Could you check a few things on this model? Use its own coordinates, in mm. A direction names the side the tool comes from. Coordinates: 2 decimals unless noted, no trailing zeros. Loops run counter-clockwise (first coordinate to the right, second up) from the corner with the lowest first, then second, coordinate; pieces in that order, holes last. Notation, with made-up numbers: M 12,-19 L 47,-19 A25 cw 47,4 Z; hole C -2,-33 d7. An arc over 180 degrees is marked long. Return JSON: item names as keys, results as strings. Group by question number.
from build123d import *

# Parameters (mm, degrees)
BOSS_EXTRUDE1_START      = -1
SKETCH1_W                = 1.7
SKETCH1_H                = 89.2
BOSS_EXTRUDE1_DEPTH      = 8.8
SKETCH4_W                = 33.7
SKETCH4_H                = 11.6
BOSS_EXTRUDE3_DEPTH      = 8.8
SERVO_HOLDER_DEPTH       = 1
SERVO_HOLDER_DEPTH_BACK  = 8.8
SKETCH3_W                = 14
SKETCH3_H                = 7
SKETCH3_R                = 1
SKETCH37_W               = 20
SKETCH37_H               = 7
BOSS_EXTRUDE19_DEPTH     = 9.8
CUT_EXTRUDE10_DEPTH      = 93.434679639
CUT_EXTRUDE10_DEPTH_BACK = 93.434679639
SKETCH29_W               = 34.409909993
SKETCH29_H               = 6.377389624
BOSS_EXTRUDE13_START     = 2
SKETCH30_W               = 34
SKETCH30_H               = 38
SKETCH30_R               = 1.6
BOSS_EXTRUDE13_DEPTH     = 6.5
SKETCH41_W               = 17.288461538
SKETCH41_H               = 8.8
CUT_EXTRUDE14_DEPTH      = 15
BOSS_EXTRUDE14_START     = -38
SKETCH32_R               = 1.45
SKETCH32_R_2             = 5
BOSS_EXTRUDE14_DEPTH     = 8.8
BOSS_EXTRUDE16_DEPTH     = 3
BOSS_EXTRUDE17_DEPTH     = 3
BOSS_EXTRUDE18_DEPTH     = 8.8
SKETCH39_W               = 1.7
SKETCH39_H               = 41.2
BOSS_EXTRUDE20_DEPTH     = 8.8
CUT_EXTRUDE13_DEPTH      = 17.5
CHAMFER2_SIZE            = 0.6
CHAMFER2_SIZE_2          = 1.039230485
CHAMFER3_SIZE            = 3
FILLET10_R               = 6
CUT_EXTRUDE15_DEPTH      = 10
CHAMFER4_SIZE            = 2.5
CUT_EXTRUDE16_DEPTH      = 10
FILLET11_R               = 0.8
SKETCH44_W               = 59.192885725
SKETCH44_H               = 45.417181718
CUT_EXTRUDE17_DEPTH      = 87.948983376


with BuildPart() as part:
    # Sketch1 → Boss-Extrude1 (new body)
    with BuildSketch(Plane(origin=(0, 0, 0), x_dir=(1, 0, 0), z_dir=(0, 1, 0)).offset(BOSS_EXTRUDE1_START)):
        with Locations((-20.85, 25.311538462)):
            Rectangle(SKETCH1_W, SKETCH1_H)
    extrude(amount=-BOSS_EXTRUDE1_DEPTH)

    # Sketch4 → Boss-Extrude3 (add)
    with BuildSketch(Plane.XZ.offset(9.8)):
        with Locations((-4.85, -64.111538462)):
            Rectangle(SKETCH4_W, SKETCH4_H)
    extrude(amount=-BOSS_EXTRUDE3_DEPTH)

    # Sketch3 → Servo Holder (add, two sides: drawn at the far end of the back side and taken through both)
    # profile 1 of 2: a face of its own
    with BuildSketch(Plane.XZ.offset(9.8).offset(-SERVO_HOLDER_DEPTH_BACK)):
        with Locations((-14.7, -55.411538462)):
            Rectangle(SKETCH3_W, SKETCH3_H)
        with Locations(Location((-14, -54.311538462, 0), (0, 0, 270))):
            Circle(SKETCH3_R, mode=Mode.SUBTRACT)
    # profile 2 of 2: a face of its own
    with BuildSketch(Plane.XZ.offset(9.8).offset(-SERVO_HOLDER_DEPTH_BACK)):
        with Locations((-14.7, -25.211538462)):
            Rectangle(SKETCH3_W, SKETCH3_H)
        with Locations(Location((-14, -26.311538462, 0), (0, 0, 90))):
            Circle(SKETCH3_R, mode=Mode.SUBTRACT)
    extrude(amount=SERVO_HOLDER_DEPTH + SERVO_HOLDER_DEPTH_BACK)

    # Sketch37 → Boss-Extrude19 (add)
    with BuildSketch(Plane(origin=(0, -1, 0), x_dir=(1, 0, 0), z_dir=(0, 1, 0))):
        with Locations((2.3, 25.211538462)):
            Rectangle(SKETCH37_W, SKETCH37_H)
    extrude(amount=-BOSS_EXTRUDE19_DEPTH)

    # Sketch29 → Cut-Extrude10 (cut, two sides: drawn at the far end of the back side and taken through both)
    with BuildSketch(Plane(origin=(0, 0, -69.911538462), x_dir=(-1, 0, 0), z_dir=(0, 0, -1)).offset(-CUT_EXTRUDE10_DEPTH_BACK)):
        with Locations((4.495045004, -12.988694812)):
            Rectangle(SKETCH29_W, SKETCH29_H)
    extrude(amount=CUT_EXTRUDE10_DEPTH + CUT_EXTRUDE10_DEPTH_BACK, mode=Mode.SUBTRACT)


with BuildPart() as body_2:
    # Sketch30 → Boss-Extrude13 (new body)
    with BuildSketch(Plane.XY.offset(BOSS_EXTRUDE13_START)):
        with Locations((-4.7, -20)):
            Rectangle(SKETCH30_W, SKETCH30_H)
        with Locations(Location((5.3, -34, 0), (0, 0, 180))):
            Circle(SKETCH30_R, mode=Mode.SUBTRACT)
        with Locations(Location((5.3, -19, 0), (0, 0, 180))):
            Circle(SKETCH30_R, mode=Mode.SUBTRACT)
        with Locations(Location((-14.7, -34, 0), (0, 0, 180))):
            Circle(SKETCH30_R, mode=Mode.SUBTRACT)
        with Locations(Location((-14.7, -19, 0), (0, 0, 180))):
            Circle(SKETCH30_R, mode=Mode.SUBTRACT)
    extrude(amount=BOSS_EXTRUDE13_DEPTH)


with BuildPart() as cut_extrude14_tool:
    # Sketch41 → Cut-Extrude14 (new body)
    with BuildSketch(Plane(origin=(-20, 0, 0), x_dir=(0, 0, -1), z_dir=(1, 0, 0))):
        with Locations((-10.644230769, -5.4)):
            Rectangle(SKETCH41_W, SKETCH41_H)
    extrude(amount=-CUT_EXTRUDE14_DEPTH)


with BuildPart() as part_1:
    add(part.part)

    # Cut-Extrude14: cut by cut_extrude14_tool
    add(cut_extrude14_tool.part, mode=Mode.SUBTRACT)



with BuildPart() as body_2_1:
    add(body_2.part)

    # Cut-Extrude14: cut by cut_extrude14_tool
    add(cut_extrude14_tool.part, mode=Mode.SUBTRACT)

    # Sketch32 → Boss-Extrude14 (add)
    with BuildSketch(Plane.XZ.offset(39).offset(BOSS_EXTRUDE14_START)):
        with BuildLine():
            ThreePointArc((11.872921748, 2), (25.925390485, -3.535644523), (35.05, 8.5))
            ThreePointArc((35.05, 8.5), (22.55, 21), (10.05, 8.5))
            Line((10.05, 8.5), (12.3, 8.5))
            Line((12.3, 8.5), (12.3, 2))
            Line((12.3, 2), (11.872921748, 2))
        make_face()
        with Locations(Location((15.25884337, 2.409923235, 0), (0, 0, 180))):
            Circle(SKETCH32_R, mode=Mode.SUBTRACT)
        with Locations(Location((28.640076765, 1.20884337, 0), (0, 0, 180))):
            Circle(SKETCH32_R, mode=Mode.SUBTRACT)
        with Locations(Location((16.459923235, 15.79115663, 0), (0, 0, 180))):
            Circle(SKETCH32_R, mode=Mode.SUBTRACT)
        with Locations(Location((22.55, 8.5, 0), (0, 0, 180))):
            Circle(SKETCH32_R_2, mode=Mode.SUBTRACT)
        with Locations(Location((29.84115663, 14.590076765, 0), (0, 0, 180))):
            Circle(SKETCH32_R, mode=Mode.SUBTRACT)
    extrude(amount=BOSS_EXTRUDE14_DEPTH)


with BuildPart() as part_2:
    add(part_1.part)

    add(body_2_1.part)  # Boss-Extrude16 merges body 2
    # Sketch34 → Boss-Extrude16 (add)
    with BuildSketch(Plane.ZY.offset(21.7)):
        Polygon((-21.711538462, -1), (-21.711538462, -9.8), (2, -39), (8.5, -39), (8.5, -1), align=None)
    extrude(amount=-BOSS_EXTRUDE16_DEPTH)

    # Sketch35 → Boss-Extrude17 (add)
    with BuildSketch(Plane(origin=(12.3, 0, 0), x_dir=(0, 0, -1), z_dir=(1, 0, 0))):
        Polygon((-2, -1), (21.711538462, -1), (21.711538462, -9.8), (-2, -39), (-8.5, -39), (-8.5, -9.8), (-8.5, -1), align=None)
    extrude(amount=-BOSS_EXTRUDE17_DEPTH)

    # Sketch36 → Boss-Extrude18 (add)
    with BuildSketch(Plane.XZ.offset(9.8)):
        Polygon((12.3, -10.579162849), (16.63422252, -2.511520186), (12.3, 1.345455989), align=None)
    extrude(amount=-BOSS_EXTRUDE18_DEPTH)

    # Sketch39 → Boss-Extrude20 (add)
    with BuildSketch(Plane(origin=(0, -1, 0), x_dir=(1, 0, 0), z_dir=(0, 1, 0))):
        with Locations((11.45, 49.311538462)):
            Rectangle(SKETCH39_W, SKETCH39_H)
    extrude(amount=-BOSS_EXTRUDE20_DEPTH)

    # Sketch40 → Cut-Extrude13 (cut)
    with BuildSketch(Plane(origin=(12.3, 0, 0), x_dir=(0, 0, -1), z_dir=(1, 0, 0))):
        Polygon((64.111538462, -1), (60.611538462, -1), (60.611538462, -2.2), (59.611538462, -2.2), (59.611538462, -6.2), (64.111538462, -6.2), align=None)
        Polygon((67.611538462, -1), (64.111538462, -1), (64.111538462, -6.2), (68.611538462, -6.2), (68.611538462, -2.2), (67.611538462, -2.2), align=None)
    extrude(amount=-CUT_EXTRUDE13_DEPTH, mode=Mode.SUBTRACT)

    # Chamfer2
    # the kernel refuses this chamfer: 1.039230485, 0.6 mm, written as the material it takes off along each edge
    with BuildSketch(Plane(origin=(14.988578382, -2.2, -67.611538462), x_dir=(0, 0.9983227437537925, 0.05789386240267319), z_dir=(-1, 0, 0))) as chamfer2_piece_1_section:
        Polygon((CHAMFER2_SIZE * 0.998322743754, CHAMFER2_SIZE * 0.0578938624027), (-CHAMFER2_SIZE_2 * 0.0578938623771, CHAMFER2_SIZE_2 * 0.998322743313), (0, 0), align=None)
    chamfer2_piece_1 = extrude(amount=20.188578382, mode=Mode.PRIVATE)
    chamfer2_piece_1 = split(chamfer2_piece_1, bisect_by=Plane(origin=(4.894289191, -2.005782009, -68.611538462), z_dir=(0, 0, 1)), keep=Keep.TOP, mode=Mode.PRIVATE)
    add(chamfer2_piece_1, mode=Mode.SUBTRACT)
    with BuildSketch(Plane(origin=(14.988578382, -2.2, -60.611538462), x_dir=(0, 0.9983227437537925, -0.05789386240267317), z_dir=(-1, 0, 0))) as chamfer2_piece_2_section:
        Polygon((CHAMFER2_SIZE * 0.998322743754, -CHAMFER2_SIZE * 0.0578938624027), (-CHAMFER2_SIZE_2 * 0.0578938623771, -CHAMFER2_SIZE_2 * 0.998322743313), (0, 0), align=None)
    chamfer2_piece_2 = extrude(amount=20.188578382, mode=Mode.PRIVATE)
    chamfer2_piece_2 = split(chamfer2_piece_2, bisect_by=Plane(origin=(4.894289191, -2.005782009, -59.611538462), z_dir=(0, 0, -1)), keep=Keep.TOP, mode=Mode.PRIVATE)
    add(chamfer2_piece_2, mode=Mode.SUBTRACT)

    # Chamfer3
    chamfer3_edges = [part_2.edges().sort_by_distance(p)[0] for p in [
        (10.6, -5.4, -58.311538462),
        (10.6, -5.4, -28.711538462),
    ]]
    chamfer(chamfer3_edges, length=CHAMFER3_SIZE)

    # Fillet10
    fillet10_edges = [part_2.edges().sort_by_distance(p)[0] for p in [
        (16.63422252, -5.4, -2.511520186),
        (12.3, -5.4, -10.579162849),
    ]]
    fillet(fillet10_edges, radius=FILLET10_R)

    # Sketch42 → Cut-Extrude15 (cut)
    with BuildSketch(Plane.XY.offset(8.5)):
        with BuildLine():
            Line((-1.1, -1), (-1.1, -10.6))
            ThreePointArc((-1.1, -10.6), (-4.7, -14.2), (-8.3, -10.6))
            Line((-8.3, -10.6), (-8.3, -1))
            Line((-8.3, -1), (-1.1, -1))
        make_face()
    extrude(amount=-CUT_EXTRUDE15_DEPTH, mode=Mode.SUBTRACT)

    # Chamfer4
    chamfer4_edges = [part_2.edges().sort_by_distance(p)[0] for p in [
        (-7.7, -5.4, -58.311538462),
    ]]
    chamfer(chamfer4_edges, length=CHAMFER4_SIZE)

    # Sketch43 → Cut-Extrude16 (cut)
    with BuildSketch(Plane(origin=(0, -1, 0), x_dir=(1, 0, 0), z_dir=(0, 1, 0))):
        Polygon((-5.2, 58.311538462), (-11.6, 51.911538462), (-5.2, 51.911538462), align=None)
    extrude(amount=-CUT_EXTRUDE16_DEPTH, mode=Mode.SUBTRACT)

    # Fillet11
    fillet11_edges = [part_2.edges().sort_by_distance(p)[0] for p in [
        (-20, -5.4, -28.711538462),
        (-20, -5.4, -51.911538462),
        (10.6, -5.4, -55.311538462),
        (10.6, -5.4, -31.711538462),
        (7.6, -5.4, -28.711538462),
        (7.6, -5.4, -58.311538462),
        (-5.2, -5.4, -58.311538462),
        (-11.6, -5.4, -51.911538462),
    ]]
    fillet(fillet11_edges, radius=FILLET11_R)

    # Sketch44 → Cut-Extrude17 (cut, through all)
    with BuildSketch(Plane(origin=(0, -1, 0), x_dir=(1, 0, 0), z_dir=(0, 1, 0))):
        with Locations((7.896442862, -0.997052397)):
            Rectangle(SKETCH44_W, SKETCH44_H)
    extrude(amount=-CUT_EXTRUDE17_DEPTH, mode=Mode.SUBTRACT)


solid = part_2.part
(1) We'd pull the mould along X, two halves only. Please class faces 4 (the face through (-20, -5, -40)), 5 (the face through (-5, -5, -69.912)), 6 (the face through (-21.7, -5, -45)), 7 (the face through (12.3, -5, -45)): +X half, -X half, draft (parallel to the pull), parting line (faces both ways), or undercut.
(2) If I drill on L1, parallel to Z at x = -14, y = -5.75; L2, parallel to Z at x = -4.5, y = -5.5; L3, parallel to Z at x = 4.5, y = -1.5, over which ranges is the centre line in solid material (lowest first)? Write a range as [from, to].
(3) Imagine slicing it at B-B, the plane x = 4. Write out the boundary of the cut face in (y, z), then the cut area to 3 significant figures.
(4) Imagine slicing it at C-C, the plane z = -54. Write out the boundary of the cut face in (x, y), then the cut area to 3 significant figures.
(5) Imagine slicing it at D-D, the plane x = -14. Write out the boundary of the cut face in (y, z).
(6) Imagine slicing it at A-A, the plane y = -3. Write out the boundary of the cut face in (x, z).
(7) Will these pins go through, and if not, where does the flat tip stop? P1, Ø10, axis at x = -2.5, z = -50.5, coming from the +Y side; P2, Ø2.5, axis at y = -3.5, z = -66.5, coming from the +X side.
(8) For faces 1 (the face through (-7, -1, -57)), 2 (the face through (4, -6.2, -64)), 3 (the face through (1, -5, -58.312)), which set-ups out of +Z, -Z, +X, -X, +Y, -Y let a thin tool reach every point of the face, with its end or its side?
Checks:
{
 "1": {"face 4": "undercut", "face 5": "draft", "face 6": "-X half", "face 7": "+X half"},
 "2": {"L1": "[-69.91, -55.31], [-53.31, -51.91], [-28.71, -27.31], [-25.31, -21.71]", "L2": "[-69.91, -68.61], [-59.61, -58.31], [-28.71, -21.71]", "L3": "[-69.91, -67.61], [-60.61, -58.31], [-28.71, -21.71]"},
 "3": {"outline": "M -9.8,-69.91 L -1,-69.91 L -1,-67.61 L -1.6,-67.61 L -2.18,-68.61 L -6.2,-68.61 L -6.2,-59.61 L -2.18,-59.61 L -1.6,-60.61 L -1,-60.61 L -1,-58.31 L -9.8,-58.31 Z; M -9.8,-28.71 L -1,-28.71 L -1,-21.71 L -9.8,-21.71 Z", "area": "119 mm²"},
 "4": {"outline": "M -21.7,-9.8 L -14.95,-9.8 L -14.95,-1 L -21.7,-1 Z; M -13.05,-9.8 L -9.51,-9.8 L -9.51,-1 L -13.05,-1 Z; M 10.6,-9.8 L 12.3,-9.8 L 12.3,-1 L 10.6,-1 Z", "area": "105 mm²"},
 "5": {"outline": "M -9.8,-69.91 L -1,-69.91 L -1,-55.31 L -9.8,-55.31 Z; M -9.8,-53.31 L -1,-53.31 L -1,-51.91 L -9.8,-51.91 Z; M -9.8,-28.71 L -1,-28.71 L -1,-27.31 L -9.8,-27.31 Z; M -9.8,-25.31 L -1,-25.31 L -1,-21.71 L -9.8,-21.71 Z"},
 "6": {"outline": "M -21.7,-69.91 L 12.3,-69.91 L 12.3,-68.61 L -5.2,-68.61 L -5.2,-59.61 L 12.3,-59.61 L 12.3,-21.71 L -21.7,-21.71 Z; hole M -20,-51.11 A0.8 ccw -19.2,-51.91 L -11.93,-51.91 A0.8 cw -11.37,-52.15 L -5.43,-58.08 A0.8 ccw -4.87,-58.31 L 7.27,-58.31 A0.8 ccw 7.83,-58.08 L 10.37,-55.55 A0.8 ccw 10.6,-54.98 L 10.6,-32.04 A0.8 ccw 10.37,-31.48 L 7.83,-28.95 A0.8 ccw 7.27,-28.71 L -19.2,-28.71 A0.8 ccw -20,-29.51 Z; hole C -14,-54.31 d2; hole C -14,-26.31 d2"},
 "7": {"P1": "through", "P2": "x = -5.2"},
 "8": {"face 1": "+Z, -Z, +X, -X, +Y", "face 2": "+X", "face 3": "+Y, -Y"}
}
